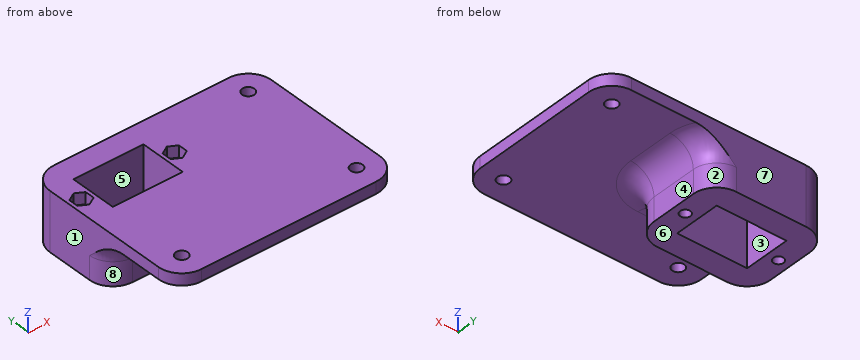
```python
from build123d import *

# Parameters (mm, degrees)
SKETCH_1_W               = 95
SKETCH_1_H               = 75
SKETCH_1_W_2             = 30
SKETCH_1_H_2             = 20
EXTRUDE_1_DEPTH          = 5
EXTRUDE_START            = -5
SKETCH_2_W               = 50
SKETCH_2_H               = 40
SKETCH_2_W_2             = 30
SKETCH_2_H_2             = 20
EXTRUDE_2_DEPTH          = 20
CUT_EXTRUDE_1_DEPTH      = 93.466210045
CUT_EXTRUDE_1_DEPTH_BACK = 93.466210045
SKETCH_3_R               = 2.2
CUT_EXTRUDE_2_DEPTH      = 5
SKETCH_5_R               = 2.6
CUT_EXTRUDE_3_DEPTH      = 93.466210045
FILLET_4_R               = 10
FILLET_5_R               = 10


with BuildPart() as part:
    # 草图1 → 凸台-拉伸1 (new body)
    with BuildSketch(Plane.XY):
        with Locations((22.5, -17.5)):
            Rectangle(SKETCH_1_W, SKETCH_1_H)
        Rectangle(SKETCH_1_W_2, SKETCH_1_H_2, mode=Mode.SUBTRACT)
    extrude(amount=EXTRUDE_1_DEPTH)

    # 草图2 → 凸台-拉伸2 (add)
    with BuildSketch(Plane.XY.offset(5).offset(EXTRUDE_START)):
        Rectangle(SKETCH_2_W, SKETCH_2_H)
        Rectangle(SKETCH_2_W_2, SKETCH_2_H_2, mode=Mode.SUBTRACT)
    extrude(amount=-EXTRUDE_2_DEPTH)

    # 草图3 → 切除-拉伸1 (cut, two sides: drawn at the far end of the back side and taken through both)
    with BuildSketch(Plane(origin=(0, 0, -20), x_dir=(-1, 0, 0), z_dir=(0, 0, -1)).offset(-CUT_EXTRUDE_1_DEPTH_BACK)):
        with Locations((20, 0)):
            Circle(SKETCH_3_R)
        with Locations((-20, 0)):
            Circle(SKETCH_3_R)
    extrude(amount=CUT_EXTRUDE_1_DEPTH + CUT_EXTRUDE_1_DEPTH_BACK, mode=Mode.SUBTRACT)

    # 草图4 → 切除-拉伸2 (cut)
    with BuildSketch(Plane(origin=(0, 0, 0), x_dir=(-1, 0, 0), z_dir=(0, 0, -1))):
        Polygon((20, 4.041451884), (16.5, 2.020725942), (16.5, -2.020725942), (20, -4.041451884), (23.5, -2.020725942), (23.5, 2.020725942), align=None)
        Polygon((-20, 4.041451884), (-23.5, 2.020725942), (-23.5, -2.020725942), (-20, -4.041451884), (-16.5, -2.020725942), (-16.5, 2.020725942), align=None)
    extrude(amount=-CUT_EXTRUDE_2_DEPTH, mode=Mode.SUBTRACT)

    # 草图5 → 切除-拉伸3 (cut, through all)
    with BuildSketch(Plane.XY.offset(5)):
        with Locations((60, -45)):
            Circle(SKETCH_5_R)
        with Locations((-15, -45)):
            Circle(SKETCH_5_R)
        with Locations((60, 10)):
            Circle(SKETCH_5_R)
    extrude(amount=-CUT_EXTRUDE_3_DEPTH, mode=Mode.SUBTRACT)

    # 圆角4
    fillet_4_edges = [part.edges().sort_by_distance(p)[0] for p in [
        (25, 20, -10),
        (25, -20, -10),
        (-25, -20, -10),
        (-25, 20, -7.5),
        (70, 20, 2.5),
        (70, -55, 2.5),
        (-25, -55, 2.5),
    ]]
    fillet(fillet_4_edges, radius=FILLET_4_R)

    # 圆角5
    # the kernel refuses this fillet: 10 mm, written as the material it adds along each edge
    with BuildSketch(Plane(origin=(15, -20, 0), x_dir=(0, 0, -1), z_dir=(-1, 0, 0))) as fillet_5_piece_1:
        with BuildLine():
            CenterArc((FILLET_5_R, FILLET_5_R), FILLET_5_R, 180, 90)
            Line((0, FILLET_5_R), (0, 0))
            Line((0, 0), (FILLET_5_R, 0))
        make_face()
    extrude(amount=30)
    with BuildSketch(Plane(origin=(25, 10, 0), x_dir=(0, 0, -1), z_dir=(0, -1, 0))) as fillet_5_piece_2:
        with BuildLine():
            CenterArc((FILLET_5_R, FILLET_5_R), FILLET_5_R, 180, 90)
            Line((0, FILLET_5_R), (0, 0))
            Line((0, 0), (FILLET_5_R, 0))
        make_face()
    extrude(amount=20)
    with BuildSketch(Plane(origin=(-15, -10, 0), x_dir=(0.801744239297648, 0.5976672776328277, 0), z_dir=(0.5976672776328277, -0.801744239297648, 0))) as fillet_5_piece_3_section:
        with BuildLine():
            CenterArc((10 + FILLET_5_R, -FILLET_5_R), FILLET_5_R, 90, 90)
            Line((10 + FILLET_5_R, 0), (10, 0))
            Line((10, 0), (10, -FILLET_5_R))
        make_face()
    fillet_5_piece_3 = revolve(axis=Axis((-15, -10, 0), (0, 0, 1)), revolution_arc=233.296989237, mode=Mode.PRIVATE)
    fillet_5_piece_3 = split(fillet_5_piece_3, bisect_by=Plane(origin=(-25, -15.925458523, -2.890503096), z_dir=(1, 0, 0)), keep=Keep.TOP, mode=Mode.PRIVATE)
    fillet_5_piece_3 = split(fillet_5_piece_3, bisect_by=Plane(origin=(-18.102265681, -5.137109304, -2.890503096), z_dir=(-0.4999999999999994, -0.866025403784439, 0)), keep=Keep.TOP, mode=Mode.PRIVATE)
    add(fillet_5_piece_3)
    with BuildSketch(Plane(origin=(15, -10, 0), x_dir=(1, 0, 0), z_dir=(0, 1, 0))) as fillet_5_piece_4:
        with BuildLine():
            CenterArc((10 + FILLET_5_R, FILLET_5_R), FILLET_5_R, 180, 90)
            Line((10 + FILLET_5_R, 0), (10, 0))
            Line((10, 0), (10, FILLET_5_R))
        make_face()
    revolve(axis=Axis((15, -10, 0), (0, 0, -1)), revolution_arc=90)
    with BuildSketch(Plane(origin=(15, 10, 0), x_dir=(-0.597667277632828, -0.8017442392976479, 0), z_dir=(0.8017442392976479, -0.597667277632828, 0))) as fillet_5_piece_5_section:
        with BuildLine():
            CenterArc((10 + FILLET_5_R, FILLET_5_R), FILLET_5_R, 180, 90)
            Line((10 + FILLET_5_R, 0), (10, 0))
            Line((10, 0), (10, FILLET_5_R))
        make_face()
    fillet_5_piece_5 = revolve(axis=Axis((15, 10, 0), (0, 0, -1)), revolution_arc=233.296989237, mode=Mode.PRIVATE)
    fillet_5_piece_5 = split(fillet_5_piece_5, bisect_by=Plane(origin=(22.499389328, 20, -3.116283122), z_dir=(0, -1, 0)), keep=Keep.TOP, mode=Mode.PRIVATE)
    fillet_5_piece_5 = split(fillet_5_piece_5, bisect_by=Plane(origin=(22.499389328, 10, -3.116283122), z_dir=(0, 1, 0)), keep=Keep.TOP, mode=Mode.PRIVATE)
    add(fillet_5_piece_5)


solid = part.part
```
Work out the finished part from the listing and answer in its coordinate system (mm). Face numbers are marked on the shaded views. A direction names the side the tool comes from. Give positions to 0.01 mm unless a question says otherwise; leave off trailing zeros. Order: outer loops, then holes, each group sorted by start corner. A loop starts at its lowest first (then second) coordinate and runs counter-clockwise, first axis right, second up. Notation, with made-up numbers: (-3.75, 1.5) - (2.25, 1.5) arc R26 ccw to (2.25, 39.5) - close; hole circle Ø2 at (50.5, -23). An arc over 180 degrees is marked (long way). One line per item, written item: value. Start each with the question number.
1. Consider line 1 (Y direction, x = 60, z = 2.4); line 2 (X direction, y = 0, z = -10.25); line 3 (Y direction, x = -0.5, z = 3). Determine where each line is inside the solid, lowest interval first.
2. Section C-C, the plane x = 14 is taken. Write down the section's boundary in (y, z), then the cut area to 3 significant figures.
3. Which of the six approach directions +Z, -Z, +X, -X, +Y, -Y give full straight-line access (tool end or side, diameter ignored) to the marked faces 1, 2, 3 and 4?
4. For a pull along Y with two mould halves and no side action, classify the marked faces 5, 6, 7 and 8 as released by +Y, released by -Y, zero draft, split by the parting line, or undercut.
5. Each of these flat-tipped pins is pushed along its axis until it touches: pin 1 Ø12 at (x, z) = (-1, -16) entering from -Y; pin 2 Ø7.5 at (x, z) = (4.5, -12.5) entering from -Y; pin 3 Ø5 at (y, z) = (-1, -15.5) entering from +X; pin 4 Ø3 at (x, y) = (60, 10) entering from +Z. Where does it stop, or does it pass through?
6. Section A-A, the plane y = 0 is taken. Write down the section's boundary in (x, z), then the cut area to 3 significant figures.
7. Section B-B, the plane z = 1 is taken. Write down the section's boundary in (x, y), then the cut area to 3 significant figures.
8. Section D-D, the plane z = -12 is taken. Write down the section's boundary in (x, y), then the cut area to 3 significant figures.
Filled sheet:
1. line 1: -55 to -47.6, -42.4 to 7.4, 12.6 to 20
1. line 2: -25 to -22.2, -17.8 to -15, 15 to 17.8, 22.2 to 25
1. line 3: -55 to -10, 10 to 20
2. outline: (-55, 0) - (-30, 0) arc R10 cw to (-20, -10) - (-20, -20) - (-10, -20) - (-10, 5) - (-55, 5) - close; (10, -20) - (20, -20) - (20, 5) - (10, 5) - close
2. area: 696 mm²
3. face 1: +Z, -Z, -X, +Y, -Y
3. face 2: -Z, +X, +Y
3. face 3: +Z, -Z
3. face 4: -Z, +X, +Y, -Y
4. face 5: undercut
4. face 6: zero draft
4. face 7: released by +Y
4. face 8: released by -Y
5. pin 1: y = -20
5. pin 2: y = -20.08
5. pin 3: x = 25
5. pin 4: through
6. outline: (-25, -20) - (-22.2, -20) - (-22.2, 0) - (-23.5, 0) - (-23.5, 5) - (-25, 5) - close; (-17.8, -20) - (-15, -20) - (-15, 5) - (-16.5, 5) - (-16.5, 0) - (-17.8, 0) - close; (15, -20) - (17.8, -20) - (17.8, 0) - (16.5, 0) - (16.5, 5) - (15, 5) - close; (22.2, -20) - (25, -20) - (25, -10) arc R10 cw to (35, 0) - (70, 0) - (70, 5) - (23.5, 5) - (23.5, 0) - (22.2, 0) - close
6. area: 500 mm²
7. outline: (-25, -45) arc R10 ccw to (-15, -55) - (60, -55) arc R10 ccw to (70, -45) - (70, 10) arc R10 ccw to (60, 20) - (-15, 20) arc R10 ccw to (-25, 10) - close; hole (-23.5, -2.02) - (-20, -4.04) - (-16.5, -2.02) - (-16.5, 2.02) - (-20, 4.04) - (-23.5, 2.02) - close; hole circle Ø5.2 at (-15, -45); hole (-15, -10) - (15, -10) - (15, 10) - (-15, 10) - close; hole (16.5, -2.02) - (20, -4.04) - (23.5, -2.02) - (23.5, 2.02) - (20, 4.04) - (16.5, 2.02) - close; hole circle Ø5.2 at (60, -45); hole circle Ø5.2 at (60, 10)
7. area: 6,290 mm²
8. outline: (-25, -10) arc R10 ccw to (-15, -20) - (15, -20) arc R10 ccw to (25, -10) - (25, 10) arc R10 ccw to (15, 20) - (-15, 20) arc R10 ccw to (-25, 10) - close; hole circle Ø4.4 at (-20, 0); hole (-15, -10) - (15, -10) - (15, 10) - (-15, 10) - close; hole circle Ø4.4 at (20, 0)
8. area: 1,280 mm²
